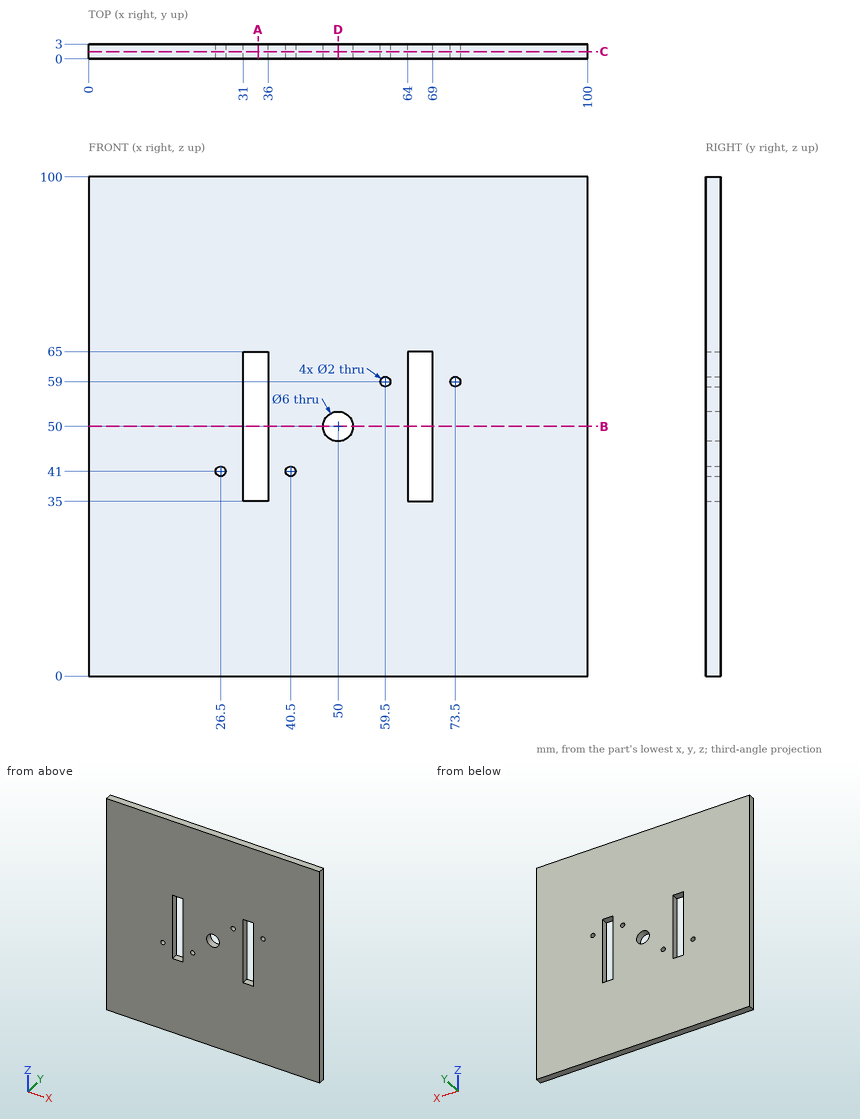
Study the drawing (mm; zero at the part's minimum x, y, z) and answer. Coordinates: 2 decimals unless noted, no trailing zeros. Loops run counter-clockwise (first coordinate to the right, second up) from the corner with the lowest first, then second, coordinate; pieces in that order, holes last. Notation, with made-up numbers: (-27.5, 39.25) -> (22.5, 39.25) arc R24 ccw to (22.5, 58.25) -> close; hole circle Ø5 at (-6, 17.5). An arc over 180 degrees is marked (long way). Answer in a Markdown table with one row per item. Add a question column.
1. The part is cut by section A-A, the plane x = 34. Write down the section's boundary in (y, z).
2. The part is cut by section D-D, the plane x = 50. Write down the section's boundary in (y, z), then the cut area to 3 significant figures.
3. The part is cut by section B-B, the plane z = 50. Write down the section's boundary in (x, y).
4. Consider line 1 (X direction, y = 1.75, z = 41); line 2 (X direction, y = 0.6, z = 64); line 3 (Z direction, x = 35, y = 1.1). Determine where each line is inside the solid, lowest interval first. Write a range as [from, to].
5. The part is cut by section C-C, the plane y = 1.45. Write down the section's boundary in (x, z), then the cut area to 3 significant figures.
Answer below:
| question | item | result |
|---|---|---|
| 1 | outline | (0, 0) -> (3, 0) -> (3, 35) -> (0, 35) -> close; (0, 65) -> (3, 65) -> (3, 100) -> (0, 100) -> close |
| 2 | outline | (0, 0) -> (3, 0) -> (3, 47) -> (0, 47) -> close; (0, 53) -> (3, 53) -> (3, 100) -> (0, 100) -> close |
| 2 | area | 282 mm2 |
| 3 | outline | (0, 0) -> (31, 0) -> (31, 3) -> (0, 3) -> close; (36, 0) -> (47, 0) -> (47, 3) -> (36, 3) -> close; (53, 0) -> (64, 0) -> (64, 3) -> (53, 3) -> close; (69, 0) -> (100, 0) -> (100, 3) -> (69, 3) -> close |
| 4 | line 1 | [0, 25.5], [27.5, 31], [36, 39.5], [41.5, 64], [69, 100] |
| 4 | line 2 | [0, 31], [36, 64], [69, 100] |
| 4 | line 3 | [0, 35], [65, 100] |
| 5 | outline | (0, 0) -> (100, 0) -> (100, 100) -> (0, 100) -> close; hole circle Ø2 at (26.5, 41); hole (31, 35) -> (36, 35) -> (36, 65) -> (31, 65) -> close; hole circle Ø2 at (40.5, 41); hole circle Ø6 at (50, 50); hole circle Ø2 at (59.5, 59); hole (64, 35) -> (69, 35) -> (69, 65) -> (64, 65) -> close; hole circle Ø2 at (73.5, 59) |
| 5 | area | 9,660 mm2 |
